Verification items for the finished model (mm, model axes). Face numbers are marked on the shaded views. A direction names the side the tool comes from. Coordinates: 2 decimals unless noted, no trailing zeros. Write each loop counter-clockwise with the first axis right and the second up, starting at its lowest first coordinate (ties: lowest second). Pieces come first, ordered by that corner, then holes. Notation, with made-up numbers: (58.5, -34) -> (100.5, -34) arc R20 ccw to (100.5, -27) -> close; hole circle Ø1 at (-14.75, 33). An arc over 180 degrees is marked (long way). Answer in a Markdown table with one row per item.
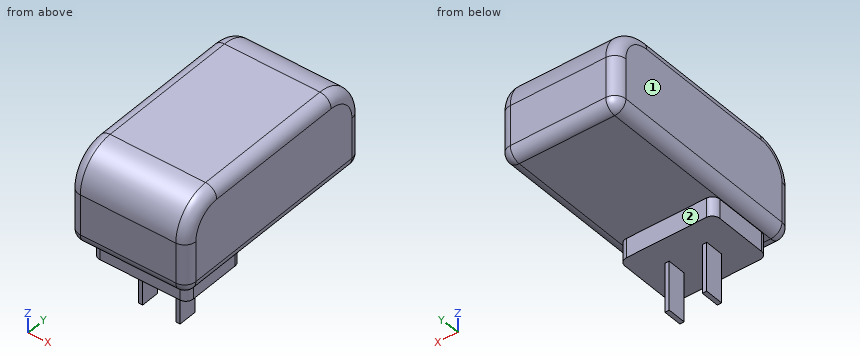
```python
from build123d import *

# Parameters (mm, degrees)
F1_DEPTH = 20.066
F2_R     = 3.81
F3_W     = 32.258
F3_H     = 22.86
F4_DEPTH = 6.604
F5_R     = 2.54
F6_W     = 1.4732
F6_H     = 6.35
F7_DEPTH = 16.764


with BuildPart() as f1:
    # F0 (on Right) → F1 (new body, symmetric)
    with BuildSketch(Plane.YZ):
        with BuildLine():
            Line((-37.084, 17.526), (-37.084, 0))
            Line((-37.084, 0), (37.084, 0))
            Line((37.084, 0), (37.084, 17.526))
            ThreePointArc((37.084, 17.526), (33.364256, 26.506256), (24.384, 30.226))
            Line((24.384, 30.226), (-24.384, 30.226))
            ThreePointArc((-24.384, 30.226), (-33.364256, 26.506256), (-37.084, 17.526))
        make_face()
    extrude(amount=F1_DEPTH, both=True)

    # F2
    f2_edges = [f1.edges().sort_by_distance(p)[0] for p in [
        (20.066, 0, 30.226),
        (-20.066, 0, 30.226),
        (0, -37.084, 0),
        (20.066, 0, 0),
        (-20.066, 0, 0),
        (0, 37.084, 0),
    ]]
    fillet(f2_edges, radius=F2_R)

    # F3 (on face) → F4 (join)
    with BuildSketch(Plane(origin=(0, 0, 0), x_dir=(1, 0, 0), z_dir=(0, 0, -1))):
        with Locations((0, 20.574)):
            Rectangle(F3_W, F3_H)
    extrude(amount=F4_DEPTH)

    # F5
    f5_edges = [f1.edges().sort_by_distance(p)[0] for p in [
        (16.129, -9.144, -3.302),
        (16.129, -32.004, -3.302),
        (-16.129, -32.004, -3.302),
        (-16.129, -9.144, -3.302),
    ]]
    fillet(f5_edges, radius=F5_R)

    # F6 (on face) → F7 (join)
    with BuildSketch(Plane(origin=(0, 0, -6.604), x_dir=(1, 0, 0), z_dir=(0, 0, -1))):
        with Locations((6.3881, 20.574)):
            Rectangle(F6_W, F6_H)
        with Locations((-6.3881, 20.574)):
            Rectangle(F6_W, F6_H)
    extrude(amount=F7_DEPTH)


solid = f1.part
```
1. Material ranges on probe 1 along X at (y, z) = (-22.5, -9.5); probe 2 along Z at (x, y) = (9, -21); probe 3 along Z at (x, y) = (-4, -8), recorded low to high. Write a range as from..to.
Findings below:
| item | result |
|---|---|
| probe 1 | x = -7.12..-5.65, 5.65..7.12 |
| probe 2 | z = -6.6..30.23 |
| probe 3 | z = 0..30.23 |
2. Go/stop test with flat-tipped pins: pin 1 (3 mm diameter, centred on y = -21.5, z = -16, fed in from -X); pin 2 (5.5 mm diameter, centred on y = -19.5, z = -5, fed in from +X); pin 3 (12 mm diameter, centred on x = 11, z = -10, fed in from -Y); pin 4 (6 mm diameter, centred on x = 6.5, z = 18.5, fed in from -Y). Record where each tip stops, or that it passes through.
Findings below:
| item | result |
|---|---|
| pin 1 | stops at x = -7.12 |
| pin 2 | stops at x = 16.13 |
| pin 3 | stops at y = -32 |
| pin 4 | stops at y = -37.08 |
3. Sectioned sample at B-B, the plane x = -3. Record the cut outline in (y, z).
Findings below:
| item | result |
|---|---|
| outline | (-37.08, 3.81) arc R3.81 ccw to (-33.27, 0) -> (-32, 0) -> (-32, -6.6) -> (-9.14, -6.6) -> (-9.14, 0) -> (33.27, 0) arc R3.81 ccw to (37.08, 3.81) -> (37.08, 17.53) arc R12.7 ccw to (24.38, 30.23) -> (-24.38, 30.23) arc R12.7 ccw to (-37.08, 17.53) -> close |
4. Sectioned sample at A-A, the plane z = -20. Record the cut outline in (x, y).
Findings below:
| item | result |
|---|---|
| outline | (-7.12, -23.75) -> (-5.65, -23.75) -> (-5.65, -17.4) -> (-7.12, -17.4) -> close; (5.65, -23.75) -> (7.12, -23.75) -> (7.12, -17.4) -> (5.65, -17.4) -> close |
5. Sectioned sample at C-C, the plane y = -8. Record the cut outline in (x, z).
Findings below:
| item | result |
|---|---|
| outline | (-20.07, 3.81) arc R3.81 ccw to (-16.26, 0) -> (16.26, 0) arc R3.81 ccw to (20.07, 3.81) -> (20.07, 26.42) arc R3.81 ccw to (16.26, 30.23) -> (-16.26, 30.23) arc R3.81 ccw to (-20.07, 26.42) -> close |
6. Access from +Z, -Z, +X, -X, +Y, -Y to the whole of each face (thin tool, end or side, straight path). Record for the marked faces 1 and 2.
Findings below:
| item | result |
|---|---|
| face 1 | +Z, -Z, -X, +Y, -Y |
| face 2 | -Z, +X, -X, +Y |
7. Sectioned sample at D-D, the plane z = -3.5. Record the cut outline in (x, y), and give its area (3 significant figures).
Findings below:
| item | result |
|---|---|
| outline | (-16.13, -29.46) arc R2.54 ccw to (-13.59, -32) -> (13.59, -32) arc R2.54 ccw to (16.13, -29.46) -> (16.13, -11.68) arc R2.54 ccw to (13.59, -9.14) -> (-13.59, -9.14) arc R2.54 ccw to (-16.13, -11.68) -> close |
| area | 732 mm² |
